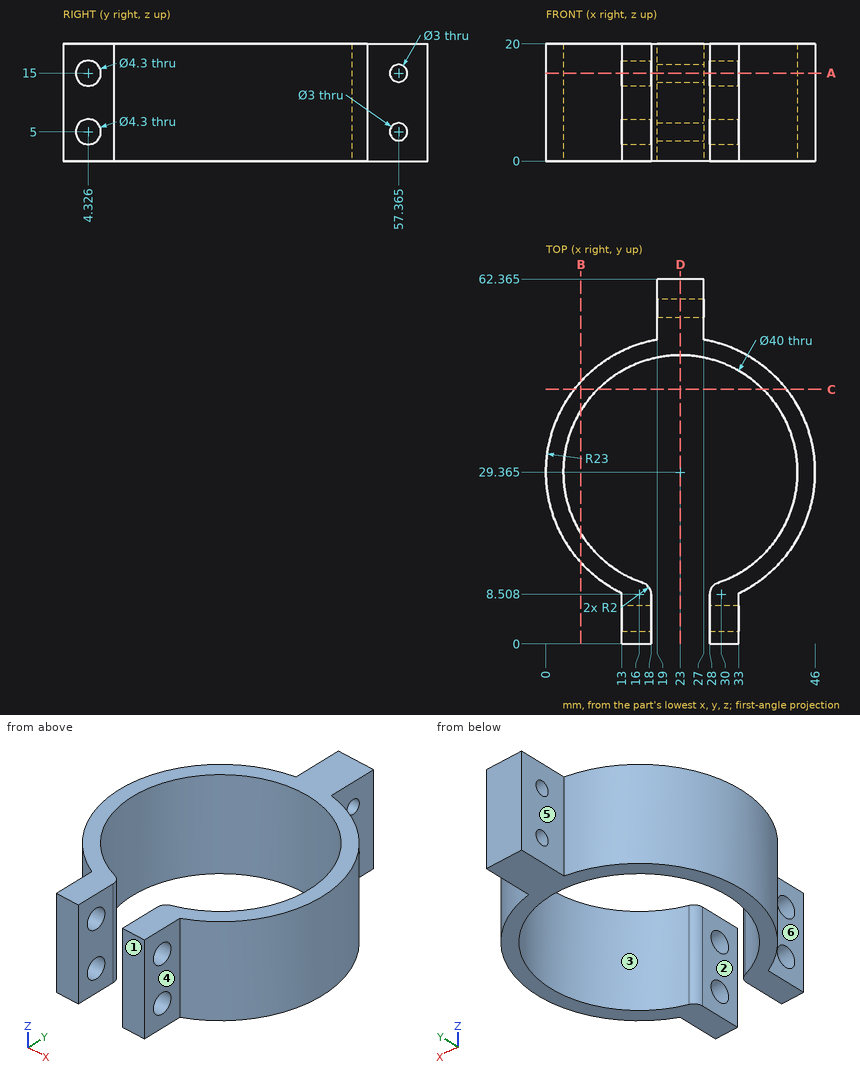
Drawing for the job (mm, zero at the part's lowest x, y, z). A direction names the side the tool comes from. Give positions to 0.01 mm unless a question says otherwise; leave off trailing zeros. Write each loop counter-clockwise with the first axis right and the second up, starting at its lowest first coordinate (ties: lowest second). Pieces come first, ordered by that corner, then holes. Notation, with made-up numbers: (40.5, 73.25) -> (45.5, 73.25) arc R26 ccw to (45.5, 95.25) -> close; hole circle Ø10 at (-36.75, 32.5). An arc over 180 degrees is marked (long way). Put each result on its own line as item: value. Start each with the question number.
Item 1: Cut at D-D (x = 23). List the corners of the cut face in (y, z) (1 decimal).
Item 2: Pull direction Y, two halves, no side cores. Call the marked faces 1, 2 and 3: pulls with the +Y half, pulls with the -Y half, needs draft (parallel to the pull), parting line crosses it, or undercut.
Item 3: Cut at A-A (z = 15). List the corners of the cut face in (x, y) (1 decimal).
Item 4: Pin check, flat tips, straight feed: pin 1 Ø9.5 at (y, z) = (4.5, 11) entering from -X; pin 2 Ø2.5 at (y, z) = (4.33, 5) entering from -X; pin 3 Ø2.5 at (y, z) = (6, 5.5) entering from +X; pin 4 Ø1.5 at (x, z) = (25, 7) entering from -Y (3 decimals). Stop position of each tip, or through.
Item 5: Cut at B-B (x = 6). List the corners of the cut face in (y, z), then the cut area to 3 significant figures.
Item 6: Cut at C-C (y = 43.5). List the corners of the cut face in (x, z), then the cut area to 3 significant figures.
Item 7: Wall check: L1, parallel to X at y = 29, z = 3.25; L2, parallel to X at y = 7, z = 16; L3, parallel to Y at x = 29, z = 12.5 (1 decimal). Give the ranges that are in metal, low to high. Write a range as [from, to].
Item 8: Which spindle directions (+Z, -Z, +X, -X, +Y, -Y) get a long thin tool onto all of the face, cutting with end or side? Do the marked faces 4, 5 and 6. Say none if no direction does.
Answer list:
1. outline: (49.4, 0) -> (62.4, 0) -> (62.4, 20) -> (49.4, 20) -> close; hole circle Ø3 at (57.4, 5); hole circle Ø3 at (57.4, 15)
2. face 1: pulls with the -Y half
2. face 2: needs draft
2. face 3: undercut
3. outline: (13, 0) -> (18, 0) -> (18, 2.2) -> (13, 2.2) -> close; (13, 6.5) -> (18, 6.5) -> (18, 8.5) arc R2 ccw to (16.6, 10.4) arc R20 cw (long way) to (29.4, 10.4) arc R2 ccw to (28, 8.5) -> (28, 6.5) -> (33, 6.5) -> (33, 8.7) arc R23 ccw to (27, 52) -> (27, 55.9) -> (19, 55.9) -> (19, 52) arc R23 ccw to (13, 8.7) -> close; (19, 58.9) -> (27, 58.9) -> (27, 62.4) -> (19, 62.4) -> close; (28, 0) -> (33, 0) -> (33, 2.2) -> (28, 2.2) -> close
4. pin 1: stops at x = 11.85
4. pin 2: passes through
4. pin 3: stops at x = 33
4. pin 4: stops at y = 49.175
5. outline: (13.87, 0) -> (18.83, 0) -> (18.83, 20) -> (13.87, 20) -> close; (39.9, 0) -> (44.86, 0) -> (44.86, 20) -> (39.9, 20) -> close
5. area: 198 mm2
6. outline: (4.86, 0) -> (8.85, 0) -> (8.85, 20) -> (4.86, 20) -> close; (37.15, 0) -> (41.14, 0) -> (41.14, 20) -> (37.15, 20) -> close
6. area: 160 mm2
7. L1: x = [0, 3], [43, 46]
7. L2: x = [13, 18], [28, 33]
7. L3: y = [0, 10.2], [48.4, 51.6]
8. face 4: +Z, -Z, +X, -Y
8. face 5: +Z, -Z, -X, +Y
8. face 6: +Z, -Z, -X, -Y
